from build123d import *

# Parameters (mm, degrees)
SKETCH1_W           = 20
SKETCH1_H           = 10
BOSS_EXTRUDE1_DEPTH = 140
SKETCH2_R           = 3
CUT_EXTRUDE1_DEPTH  = 140
LPATTERN1_COUNT     = 4
LPATTERN1_PITCH     = 40


with BuildPart() as part:
    # Sketch1 → Boss-Extrude1 (new body)
    with BuildSketch(Plane.XY):
        with Locations((10, 15.187969925)):
            Rectangle(SKETCH1_W, SKETCH1_H)
    extrude(amount=BOSS_EXTRUDE1_DEPTH)

    # Sketch2 → Cut-Extrude1 (cut)
    with BuildSketch(Plane(origin=(0, 20.187969925, 0), x_dir=(1, 0, 0), z_dir=(0, 1, 0))):
        with Locations((14.108562183, -8.673667423)):
            Circle(SKETCH2_R)
    cut_extrude1 = extrude(amount=-CUT_EXTRUDE1_DEPTH, mode=Mode.SUBTRACT)

    # LPattern1: Cut-Extrude1 ×4
    with Locations(*[(0, 0, i * LPATTERN1_PITCH) for i in range(1, LPATTERN1_COUNT)]):
        add(cut_extrude1, mode=Mode.SUBTRACT)


solid = part.part
Build history of the part. All positions in model axes, mm. Give positions to 0.01 mm unless a question says otherwise; leave off trailing zeros. Write each loop counter-clockwise with the first axis right and the second up, starting at its lowest first coordinate (ties: lowest second). Pieces come first, ordered by that corner, then holes. Notation, with made-up numbers: (65, 27) - (89, 27) arc R18 ccw to (89, 51) - close; hole circle Ø4 at (89, 74). An arc over 180 degrees is marked (long way). Use one line per item in the form item = value. Start each with the question number.
1. Band-saw the part on B-B on y = 12. Write the cut outline in (x, z).
2. Band-saw the part on A-A on x = 15.5. Write the cut outline in (y, z), plus the area to 3 significant figures.
3. Probe line 1 (Z direction, x = 15, y = 19.25); line 2 (Z direction, x = 11.5, y = 12.5); line 3 (X direction, y = 16, z = 11). List the from-to ranges inside material, lowest first. Write a range as [from, to].
4. Two-plate mould, pull along Z, no slides. Class faces 1 (the face through (0, 15, 69)), 2 (the face through (10, 15, 0)), 3 (the face through (13.458, 15.258, 131.602)), 4 (the face through (10, 15, 140)): released by +Z, released by -Z, zero draft, split by the parting line, or undercut.
Conclusion:
q1.outline = (0, 0) - (20, 0) - (20, 140) - (0, 140) - close; hole circle Ø6 at (14.11, 8.67); hole circle Ø6 at (14.11, 48.67); hole circle Ø6 at (14.11, 88.67); hole circle Ø6 at (14.11, 128.67)
q2.outline = (10.19, 0) - (20.19, 0) - (20.19, 6.02) - (10.19, 6.02) - close; (10.19, 11.33) - (20.19, 11.33) - (20.19, 46.02) - (10.19, 46.02) - close; (10.19, 51.33) - (20.19, 51.33) - (20.19, 86.02) - (10.19, 86.02) - close; (10.19, 91.33) - (20.19, 91.33) - (20.19, 126.02) - (10.19, 126.02) - close; (10.19, 131.33) - (20.19, 131.33) - (20.19, 140) - (10.19, 140) - close
q2.area = 1,190 mm²
q3.line_1 = [0, 5.81], [11.54, 45.81], [51.54, 85.81], [91.54, 125.81], [131.54, 140]
q3.line_2 = [0, 7.19], [10.16, 47.19], [50.16, 87.19], [90.16, 127.19], [130.16, 140]
q3.line_3 = [0, 12.21], [16, 20]
q4.face_1 = zero draft
q4.face_2 = released by -Z
q4.face_3 = undercut
q4.face_4 = released by +Z
